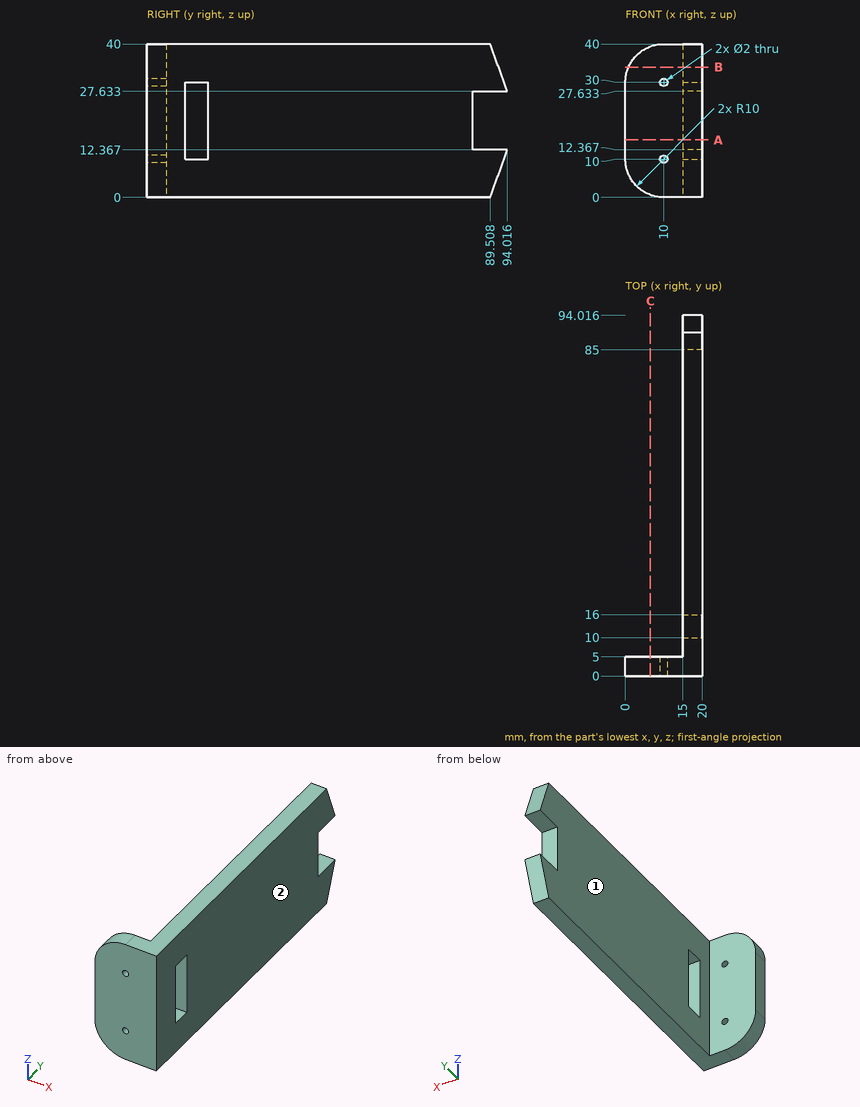
Answer from the drawing. Dimensions are ordinates in mm from the lowest x, y and z of the part. A direction names the side the tool comes from. Coordinates: 2 decimals unless noted, no trailing zeros. Write each loop counter-clockwise with the first axis right and the second up, starting at its lowest first coordinate (ties: lowest second). Pieces come first, ordered by that corner, then holes. Notation, with made-up numbers: M 28.5,9.5 L 36.5,9.5 A13 ccw 36.5,21.5 Z; hole C 20.25,48 d3. An arc over 180 degrees is marked long. Put each result on its own line as item: value. Start each with the question number.
1. A cutting plane is placed at A-A on z = 15. Write down the section's boundary in (x, y), then the cut area to 3 significant figures.
2. A cutting plane is placed at C-C on x = 6.5. Write down the section's boundary in (y, z).
3. Which of the six approach directions +Z, -Z, +X, -X, +Y, -Y give full straight-line access (tool end or side, diameter ignored) to the marked faces 1 and 2?
4. Flat-ended cylindrical pins translate along their axes: P1, Ø5.5, axis at x = 18.5, z = 17, coming from the +Y side; P2, Ø4, axis at x = 4.5, z = 7.5, coming from the -Y side; P3, Ø3, axis at x = 10, z = 30, coming from the +Y side; P4, Ø20, axis at y = 46, z = 24, coming from the -X side. Find the tip coordinate at first contact, or state that the pin passes through.
5. Consider line 1 (Z direction, x = 10, y = 3.7); line 2 (X direction, y = 1.5, z = 30); line 3 (Y direction, x = 16, z = 16). Determine where each line is inside the solid, lowest interval first. Write a range as from..to.
6. A cutting plane is placed at B-B on z = 34. Write down the section's boundary in (x, y) (1 decimal).
Resolved:
1. outline: M 0,0 L 20,0 L 20,10 L 15,10 L 15,5 L 0,5 Z; M 15,16 L 20,16 L 20,85 L 15,85 Z
1. area: 470 mm2
2. outline: M 0,0.63 L 5,0.63 L 5,39.37 L 0,39.37 Z
3. face 1: +Z, -Z, -X, +Y
3. face 2: +Z, -Z, +X, +Y, -Y
4. P1: stops at y = 85
4. P2: stops at y = 0
4. P3: stops at y = 5
4. P4: stops at x = 15
5. line 1: z = 0..9, 11..29, 31..40
5. line 2: x = 0..9, 11..20
5. line 3: y = 0..10, 16..85
6. outline: M 0.8,0 L 20,0 L 20,91.7 L 15,91.7 L 15,5 L 0.8,5 Z
